Build history of the part. All positions in model axes, mm. A direction names the side the tool comes from. Give positions to 0.01 mm unless a question says otherwise; leave off trailing zeros. Order: outer loops, then holes, each group sorted by start corner. A loop starts at its lowest first (then second) coordinate and runs counter-clockwise, first axis right, second up. Notation, with made-up numbers: M 4,44 L 61,44 A29 cw 61,81 Z; hole C -22.5,52 d3. An arc over 180 degrees is marked long. One line per item, written item: value.
from build123d import *

# Parameters (mm, degrees)
SKETCH1_W            = 70
SKETCH1_H            = 11.5
BOSS_EXTRUDE1_DEPTH  = 20
CUT_EXTRUDE1_REACH   = 55.461
CUT_EXTRUDE2_DEPTH   = 5
HOLE1_D              = 4.5
LPATTERN1_COUNT      = 2
LPATTERN1_PITCH      = 60
LPATTERN1_COUNT_DIR2 = 2
LPATTERN1_PITCH_DIR2 = 15
HOLE2_D              = 4.5


with BuildPart() as part:
    # Sketch1 → Boss-Extrude1 (new, symmetric)
    with BuildSketch(Plane.XY):
        Rectangle(SKETCH1_W, SKETCH1_H)
    extrude(amount=BOSS_EXTRUDE1_DEPTH, both=True)

    # Sketch2 → Cut-Extrude1 (cut, up to next)
    with BuildSketch(Plane.XY.offset(20), mode=Mode.PRIVATE) as cut_extrude1_sk1:
        with BuildLine():
            Line((-25, -5.75), (-10, -5.75))
            ThreePointArc((-10, -5.75), (-17.5, 1.75), (-25, -5.75))
        make_face()
    cut_extrude1_tool1 = extrude(cut_extrude1_sk1.sketch, amount=-CUT_EXTRUDE1_REACH, mode=Mode.PRIVATE) & part.part
    # Sketch2 → Cut-Extrude1 (cut, up to next)
    with BuildSketch(Plane.XY.offset(20), mode=Mode.PRIVATE) as cut_extrude1_sk2:
        with BuildLine():
            Line((10, -5.75), (25, -5.75))
            ThreePointArc((25, -5.75), (17.5, 1.75), (10, -5.75))
        make_face()
    cut_extrude1_tool2 = extrude(cut_extrude1_sk2.sketch, amount=-CUT_EXTRUDE1_REACH, mode=Mode.PRIVATE) & part.part
    add(cut_extrude1_tool1.solids().sort_by_distance((-17.5, -2.566901, 20))[0], mode=Mode.SUBTRACT)
    add(cut_extrude1_tool2.solids().sort_by_distance((17.5, -2.566901, 20))[0], mode=Mode.SUBTRACT)

    # Sketch3 → Cut-Extrude2 (cut)
    with BuildSketch(Plane.XY.offset(20)):
        with BuildLine():
            Line((-35, 5.75), (-35, -5.75))
            Line((-35, -5.75), (-29, -5.75))
            ThreePointArc((-29, -5.75), (-25.631727984, 2.381727984), (-17.5, 5.75))
            Line((-17.5, 5.75), (-35, 5.75))
        make_face()
        with BuildLine():
            Line((29, -5.75), (35, -5.75))
            Line((35, -5.75), (35, 5.75))
            Line((35, 5.75), (17.5, 5.75))
            ThreePointArc((17.5, 5.75), (25.631727984, 2.381727984), (29, -5.75))
        make_face()
    cut_extrude2 = extrude(amount=-CUT_EXTRUDE2_DEPTH, mode=Mode.SUBTRACT)

    # Mirror1: Cut-Extrude2 across plane
    add(cut_extrude2.mirror(Plane.XY), mode=Mode.SUBTRACT)

    # Hole1 (through all)
    with Locations(Plane(origin=(0, 5.75, 0), x_dir=(1, 0, 0), z_dir=(0, 1, 0))):
        with Locations((30, -7.5)):
            hole1 = Hole(HOLE1_D / 2)

    # LPattern1: Hole1 2 × 2
    with Locations(*[(-i * LPATTERN1_PITCH, 0, -j * LPATTERN1_PITCH_DIR2) for i in range(LPATTERN1_COUNT) for j in range(LPATTERN1_COUNT_DIR2) if (i, j) != (0, 0)]):
        add(hole1, mode=Mode.SUBTRACT)

    # Hole2 (through all)
    with Locations(Plane(origin=(0, 5.75, 0), x_dir=(1, 0, 0), z_dir=(0, 1, 0))):
        with Locations((0, -15)):
            hole2 = Hole(HOLE2_D / 2)

    # Mirror2: Hole2 across plane
    add(hole2.mirror(Plane.XY), mode=Mode.SUBTRACT)


solid = part.part
1) Saw through at A-A, the plane x = 0. Write the cut outline in (y, z), then the cut area to 4 significant figures.
Check values:
outline: M -5.75,-20 L 5.75,-20 L 5.75,-17.25 L -5.75,-17.25 Z; M -5.75,-12.75 L 5.75,-12.75 L 5.75,12.75 L -5.75,12.75 Z; M -5.75,17.25 L 5.75,17.25 L 5.75,20 L -5.75,20 Z
area: 356.5 mm^2
2) Drill centre lines: probe 1 along Z at (x, y) = (0, 0.5); probe 2 along Z at (x, y) = (30, 2.5); probe 3 along X at (y, z) = (-3.25, 10). Where is each one in solid material? Low to high. Write a range as from..to.
Check values:
probe 1: -20..-17.25, -12.75..12.75, 17.25..20
probe 2: -15..-9.75, -5.25..5.25, 9.75..15
probe 3: -35..-24.57, -10.43..10.43, 24.57..35
3) Saw through at B-B, the plane z = -2.5. Write the cut outline in (x, y), then the cut area to 3 significant figures.
Check values:
outline: M -35,-5.75 L -25,-5.75 A7.5 cw -10,-5.75 L 10,-5.75 A7.5 cw 25,-5.75 L 35,-5.75 L 35,5.75 L -35,5.75 Z
area: 628 mm^2
4) Pin check, flat tip, straight feed: pin 1 (2.5 mm diameter, centred on x = -30, z = 7.5, fed in from -Y). Stop position of the tip, or through.
Check values:
pin 1: through
5) Saw through at D-D, the plane y = 3. Write the cut outline in (x, z), then the cut area to 3 significant figures.
Check values:
outline: M -35,-15 L -24.96,-15 L -24.96,-20 L 24.96,-20 L 24.96,-15 L 35,-15 L 35,15 L 24.96,15 L 24.96,20 L -24.96,20 L -24.96,15 L -35,15 Z; hole C -30,-7.5 d4.5; hole C -30,7.5 d4.5; hole C 0,-15 d4.5; hole C 0,15 d4.5; hole C 30,-7.5 d4.5; hole C 30,7.5 d4.5
area: 2,500 mm^2
6) Saw through at C-C, the plane x = -30. Write the cut outline in (y, z), then the cut area to 4 significant figures.
Check values:
outline: M -5.75,-15 L 5.75,-15 L 5.75,-9.75 L -5.75,-9.75 Z; M -5.75,-5.25 L 5.75,-5.25 L 5.75,5.25 L -5.75,5.25 Z; M -5.75,9.75 L 5.75,9.75 L 5.75,15 L -5.75,15 Z
area: 241.5 mm^2
7) Tool access for faces 4 (the face through (25.54, 2.47, -17.54)), 5 (the face through (-30, 1, -15)), 6 (the face through (30, 1, 15)): list every direction of +Z, -Z, +X, -X, +Y, -Y with a clear straight run to the whole face (end or side of a thin tool).
Check values:
face 4: -Z, +X, +Y
face 5: -Z, -X, +Y
face 6: +Z, +X, +Y
8) Mould opens along Z. For faces 1 (the face through (30, 1, -15)), 2 (the face through (17.66, 1.75, 0.28)), 3 (the face through (-31.21, -0.081, 5.603)) say: released by +Z, released by -Z, zero draft, split by the parting line, or undercut.
Check values:
face 1: released by -Z
face 2: zero draft
face 3: undercut
